Verification items for the finished model (mm, model axes). Coordinates: 2 decimals unless noted, no trailing zeros. Write each loop counter-clockwise with the first axis right and the second up, starting at its lowest first coordinate (ties: lowest second). Pieces come first, ordered by that corner, then holes. Notation, with made-up numbers: (-13.75, 81) -> (36.25, 81) arc R18 ccw to (36.25, 89) -> close; hole circle Ø1 at (-19.5, 60.5). An arc over 180 degrees is marked (long way). Write each question's results on one line, items separated by ' | '. Start each with the question number.
from build123d import *

# Parameters (mm, degrees)
F1_DEPTH = 68.97317
F2_R     = 5.08


with BuildPart() as f1:
    # F0 (on Top) → F1 (new body)
    with BuildSketch(Plane.XY):
        Polygon((0, 0), (143.774033, 7.85425), (154.337034, 85.148476), (-10.384366, 85.148476), align=None)
    extrude(amount=F1_DEPTH)

    # F2
    f2_edges = [f1.edges().sort_by_distance(p)[0] for p in [
        (-10.384366, 85.148476, 34.486585),
        (0, 0, 34.486585),
        (-5.192183, 42.574238, 0),
        (-5.192183, 42.574238, 68.97317),
        (71.976334, 85.148476, 68.97317),
        (71.887016, 3.927125, 68.97317),
        (149.055533, 46.501363, 68.97317),
    ]]
    fillet(f2_edges, radius=F2_R)


solid = f1.part
1. Sectioned sample at A-A on z = 27. Record the cut outline in (x, y).
2. Depth check by flat-ended pin: pin 1 Ø12 at (y, z) = (68.5, 41.5) entering from +X; pin 2 Ø1 at (x, z) = (122, 49) entering from -Y; pin 3 Ø1.5 at (y, z) = (55.5, 25.5) entering from +X. Enter the tip coordinate at first touch or a pass-through.
3. Material ranges on probe 1 along Y at (x, z) = (86, 38); probe 2 along Z at (x, y) = (-2.5, 44); probe 3 along X at (y, z) = (16, 22), recorded low to high. Write a range as from..to.
Computed values:
1) outline: (-9.69, 79.45) -> (-0.58, 4.72) arc R5.08 ccw to (4.74, 0.26) -> (143.77, 7.85) -> (154.34, 85.15) -> (-4.65, 85.15) arc R5.08 ccw to start
2) pin 1: stops at x = 152.88 | pin 2: stops at y = 6.64 | pin 3: stops at x = 150.39
3) probe 1: y = 4.7..85.15 | probe 2: z = 0.52..68.46 | probe 3: x = -1.95..144.89
